from build123d import *

# Parameters (mm, degrees)
SKETCH1_W           = 12
SKETCH1_H           = 6
SKETCH1_W_2         = 223
BOSS_EXTRUDE1_DEPTH = 6


with BuildPart() as part:
    # Sketch1 → Boss-Extrude1 (new body)
    with BuildSketch(Plane.XY):
        with Locations((-93.5, 6)):
            Rectangle(SKETCH1_W, SKETCH1_H)
        Rectangle(SKETCH1_W_2, SKETCH1_H)
        with Locations((0, 6)):
            Rectangle(SKETCH1_W, SKETCH1_H)
        with Locations((93.5, 6)):
            Rectangle(SKETCH1_W, SKETCH1_H)
    extrude(amount=-BOSS_EXTRUDE1_DEPTH)


solid = part.part
Could you check a few things on this model? Use its own coordinates, in mm. A direction names the side the tool comes from. Give positions to 0.01 mm unless a question says otherwise; leave off trailing zeros. Loops run counter-clockwise (first coordinate to the right, second up) from the corner with the lowest first, then second, coordinate; pieces in that order, holes last. Notation, with made-up numbers: (71, -29) -> (99, -29) arc R25 cw to (99, -6) -> close; hole circle Ø4 at (8.25, -35). An arc over 180 degrees is marked (long way). Answer as CSV lines item,"result". Start each with the question number.
(1) If we section it at B-B on z = -4.4: Write out the boundary of the cut face in (x, y), then the cut area to 3 significant figures.
(2) I'm going to push flat-ended pins straight in: pin 1 Ø1.8 at (x, z) = (-50.5, -3) entering from +Y; pin 2 Ø1.8 at (y, z) = (5.5, -2) entering from +X; pin 3 Ø1.8 at (y, z) = (5.5, -2.5) entering from -X. Where does each tip first touch, or does it pass through?
(3) I need wall thicknesses on probe 1 along X at (y, z) = (3.5, -1); probe 2 along Y at (x, z) = (-86, -5.3). Which ranges of each line are inside material? Lowest first, please.
(4) If we section it at A-A on y = 6.75: Write out the boundary of the cut face in (x, z), then the cut area to 3 significant figures.
(5) Which directions (+Z, -Z, +X, -X, +Y, -Y) give clear straight access to the entire face, cutting with the end or side of a thin tool? Please do faces 1 (the flat face through (-106, 3, -3)), 2 (the flat face through (0, 9, -3)), 3 (the flat face through (-111.5, 0, -3)), 4 (the flat face through (46, 3, -3)), 5 (the flat face through (99.5, 6, -3)).
(6) If we section it at C-C on x = 50: Write out the boundary of the cut face in (y, z), then the cut area to 3 significant figures.
Computed:
1,outline,"(-111.5, -3) -> (111.5, -3) -> (111.5, 3) -> (99.5, 3) -> (99.5, 9) -> (87.5, 9) -> (87.5, 3) -> (6, 3) -> (6, 9) -> (-6, 9) -> (-6, 3) -> (-87.5, 3) -> (-87.5, 9) -> (-99.5, 9) -> (-99.5, 3) -> (-111.5, 3) -> close"
1,area,"1,550 mm2"
2,pin 1,"stops at y = 3"
2,pin 2,"stops at x = 99.5"
2,pin 3,"stops at x = -99.5"
3,probe 1,"x = -99.5 to -87.5, -6 to 6, 87.5 to 99.5"
3,probe 2,"y = -3 to 3"
4,outline,"(-99.5, -6) -> (-87.5, -6) -> (-87.5, 0) -> (-99.5, 0) -> close; (-6, -6) -> (6, -6) -> (6, 0) -> (-6, 0) -> close; (87.5, -6) -> (99.5, -6) -> (99.5, 0) -> (87.5, 0) -> close"
4,area,"216 mm2"
5,face 1,"+Z, -Z, -X, +Y"
5,face 2,"+Z, -Z, +X, -X, +Y"
5,face 3,"+Z, -Z, -X, +Y, -Y"
5,face 4,"+Z, -Z, +Y"
5,face 5,"+Z, -Z, +X, +Y"
6,outline,"(-3, -6) -> (3, -6) -> (3, 0) -> (-3, 0) -> close"
6,area,"36.0 mm2"
